Read the model definition and answer for the solid it produces. Units are mm, in the model's axes. Face numbers are marked on the shaded views. A direction names the side the tool comes from. Round coordinates to 2 decimals unless told otherwise and drop trailing zeros. Loops run counter-clockwise (first coordinate to the right, second up) from the corner with the lowest first, then second, coordinate; pieces in that order, holes last. Notation, with made-up numbers: M 64,11.5 L 118,11.5 A26 cw 118,46.5 Z; hole C 0.5,8 d6. An arc over 180 degrees is marked long. Answer as CSV lines item,"result".
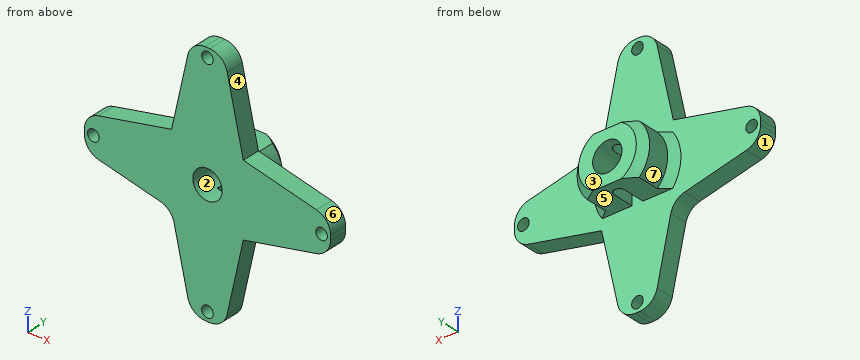
```python
from build123d import *

# Parameters (mm, degrees)
SKETCH1_R           = 34
SKETCH1_R_2         = 1.6
SKETCH1_R_3         = 4.05
BOSS_EXTRUDE1_DEPTH = 5
SKETCH2_R           = 4.05
BOSS_EXTRUDE2_DEPTH = 10
CUT_EXTRUDE1_DEPTH  = 42
CUT_EXTRUDE2_DEPTH  = 10
FILLET1_R           = 5
CHAMFER2_SIZE       = 2


with BuildPart() as part:
    # Sketch1 → Boss-Extrude1 (new body)
    with BuildSketch(Plane(origin=(0, 0, 0), x_dir=(1, 0, 0), z_dir=(0, 1, 0))):
        Circle(SKETCH1_R)
        with Locations((0, 31.5)):
            Circle(SKETCH1_R_2, mode=Mode.SUBTRACT)
        with Locations((31.5, 0)):
            Circle(SKETCH1_R_2, mode=Mode.SUBTRACT)
        with Locations((0, -31.5)):
            Circle(SKETCH1_R_2, mode=Mode.SUBTRACT)
        with Locations((-31.5, 0)):
            Circle(SKETCH1_R_2, mode=Mode.SUBTRACT)
        Circle(SKETCH1_R_3, mode=Mode.SUBTRACT)
    extrude(amount=BOSS_EXTRUDE1_DEPTH)

    # Sketch2 → Boss-Extrude2 (add)
    with BuildSketch(Plane(origin=(0, 5, 0), x_dir=(1, 0, 0), z_dir=(0, 1, 0))):
        with BuildLine():
            Line((-7.141428429, 7), (7.141428429, 7))
            ThreePointArc((7.141428429, 7), (10, 0), (7.141428429, -7))
            Line((7.141428429, -7), (-7.141428429, -7))
            ThreePointArc((-7.141428429, -7), (-10, 0), (-7.141428429, 7))
        make_face()
        Circle(SKETCH2_R, mode=Mode.SUBTRACT)
    extrude(amount=BOSS_EXTRUDE2_DEPTH)

    # Sketch3 → Cut-Extrude1 (cut, through all)
    with BuildSketch(Plane(origin=(0, 0, -7), x_dir=(-1, 0, 0), z_dir=(0, 0, -1))):
        with BuildLine():
            Line((1.5, 5), (1.5, 11))
            ThreePointArc((1.5, 11), (0, 12.5), (-1.5, 11))
            Line((-1.5, 11), (-1.5, 5))
            Line((-1.5, 5), (1.5, 5))
        make_face()
    extrude(amount=-CUT_EXTRUDE1_DEPTH, mode=Mode.SUBTRACT)

    # Sketch4 → Cut-Extrude2 (cut)
    with BuildSketch(Plane(origin=(0, 5, 0), x_dir=(1, 0, 0), z_dir=(0, 1, 0))):
        with BuildLine():
            Line((-33.682156271, 4.638140673), (-9.899494937, 9.899494937))
            Line((-9.899494937, 9.899494937), (-4.638140673, 33.682156271))
            ThreePointArc((-4.638140673, 33.682156271), (-24.04163056, 24.04163056), (-33.682156271, 4.638140673))
        make_face()
        with BuildLine():
            Line((4.638140673, 33.682156271), (9.899494937, 9.899494937))
            Line((9.899494937, 9.899494937), (33.682156271, 4.638140673))
            ThreePointArc((33.682156271, 4.638140673), (24.04163056, 24.04163056), (4.638140673, 33.682156271))
        make_face()
        with BuildLine():
            Line((33.682156271, -4.638140673), (9.899494937, -9.899494937))
            Line((9.899494937, -9.899494937), (4.638140673, -33.682156271))
            ThreePointArc((4.638140673, -33.682156271), (24.04163056, -24.04163056), (33.682156271, -4.638140673))
        make_face()
        with BuildLine():
            Line((-4.638140673, -33.682156271), (-9.899494937, -9.899494937))
            Line((-9.899494937, -9.899494937), (-33.682156271, -4.638140673))
            ThreePointArc((-33.682156271, -4.638140673), (-24.04163056, -24.04163056), (-4.638140673, -33.682156271))
        make_face()
    extrude(amount=-CUT_EXTRUDE2_DEPTH, mode=Mode.SUBTRACT)

    # Fillet1
    fillet1_edges = [part.edges().sort_by_distance(p)[0] for p in [
        (-9.899494937, 2.5, -9.899494937),
        (-33.682156271, 2.5, -4.638140673),
        (-4.638140673, 2.5, -33.682156271),
        (4.638140673, 2.5, -33.682156271),
        (33.682156271, 2.5, -4.638140673),
        (33.682156271, 2.5, 4.638140673),
        (4.638140673, 2.5, 33.682156271),
        (-4.638140673, 2.5, 33.682156271),
        (-33.682156271, 2.5, 4.638140673),
    ]]
    fillet(fillet1_edges, radius=FILLET1_R)

    # Chamfer2
    chamfer2_edges = [part.edges().sort_by_distance(p)[0] for p in [
        (-10, 15, 0),
        (10, 15, 0),
        (-10, 5, 0),
        (10, 5, 0),
    ]]
    chamfer(chamfer2_edges, length=CHAMFER2_SIZE)


solid = part.part
```
1) Find section B-B, the plane x = 31.5. Give the vertices of the cut face in (y, z), then the cut area to 3 significant figures.
Evaluation:
outline,"M 0,-4.88 L 5,-4.88 L 5,-1.6 L 0,-1.6 Z; M 0,1.6 L 5,1.6 L 5,4.88 L 0,4.88 Z"
area,"32.8 mm^2"
2) Find section A-A, the plane y = 8. Give the vertices of the cut face in (x, z).
Evaluation:
outline,"M -7.14,-7 L -1.5,-7 L -1.5,-3.76 A4.05 cw -1.5,3.76 L -1.5,7 L -7.14,7 A10 ccw Z; M 1.5,-7 L 7.14,-7 A10 ccw 7.14,7 L 1.5,7 L 1.5,3.76 A4.05 cw 1.5,-3.76 Z"
3) Each of these flat-tipped pins is pushed along its axis until it touches: P1, Ø3.5, axis at y = 9.5, z = 6, coming from the +X side; P2, Ø2.5, axis at x = -31.5, z = 0, coming from the +Y side; P3, Ø3.5, axis at y = 8, z = 6, coming from the -X side; P4, Ø6, axis at x = -8, z = 17, coming from the +Y side. Where does it stop, or does it pass through?
Evaluation:
P1,"stops at x = 9.05"
P2,"passes through"
P3,"stops at x = -9.19"
P4,"stops at y = 5"
4) A tool of negligible diameter and unlimited length cuts with its end or side. For the marked faces 5, 6 and 7, from which of +Z, -Z, +X, -X, +Y, -Y can it reach the whole face along a straight path? Write none if from no direction.
Evaluation:
face 5,"-Z, +X, -X, +Y"
face 6,"+Z, +X, +Y, -Y"
face 7,"-X, +Y"
5) Determine the mould class of the marked faces 1, 2, 3 and 4 for opening direction X: released by +X, released by -X, zero draft, split by the parting line, or undercut.
Evaluation:
face 1,"released by -X"
face 2,"undercut"
face 3,"zero draft"
face 4,"released by +X"
6) Find section D-D, the plane y = 3.5. Give the vertices of the cut face in (x, z), then the cut area to 3 significant figures.
Evaluation:
outline,"M -33.99,-0.65 A5 ccw -30.07,-5.44 L -13.01,-9.21 A5 cw -9.21,-13.01 L -5.44,-30.07 A5 ccw -0.65,-33.99 A34 ccw 0.65,-33.99 A5 ccw 5.44,-30.07 L 9.9,-9.9 L 30.07,-5.44 A5 ccw 33.99,-0.65 A34 ccw 33.99,0.65 A5 ccw 30.07,5.44 L 9.9,9.9 L 5.44,30.07 A5 ccw 0.65,33.99 A34 ccw -0.65,33.99 A5 ccw -5.44,30.07 L -9.9,9.9 L -30.07,5.44 A5 ccw -33.99,0.65 A34 ccw Z; hole C -31.5,0 d3.2; hole C 0,0 d8.1; hole C 0,-31.5 d3.2; hole C 0,31.5 d3.2; hole C 31.5,0 d3.2"
area,"1,680 mm^2"
7) Find section C-C, the plane z = 31.5. Give the vertices of the cut face in (x, y).
Evaluation:
outline,"M -4.88,0 L -1.6,0 L -1.6,5 L -4.88,5 Z; M 1.6,0 L 4.88,0 L 4.88,5 L 1.6,5 Z"
8) Straight lines are drawn through the part: line 1 (Z direction, x = 0, y = 1.1); line 2 (Y direction, x = -16.5, z = 3); line 3 (Z direction, x = -31.5, y = 3.6). For each, find the intervals that lie inside material, in ascending order.
Evaluation:
line 1,"z = -34 to -33.1, -29.9 to -4.05, 4.05 to 29.9, 33.1 to 34"
line 2,"y = 0 to 5"
line 3,"z = -4.88 to -1.6, 1.6 to 4.88"
